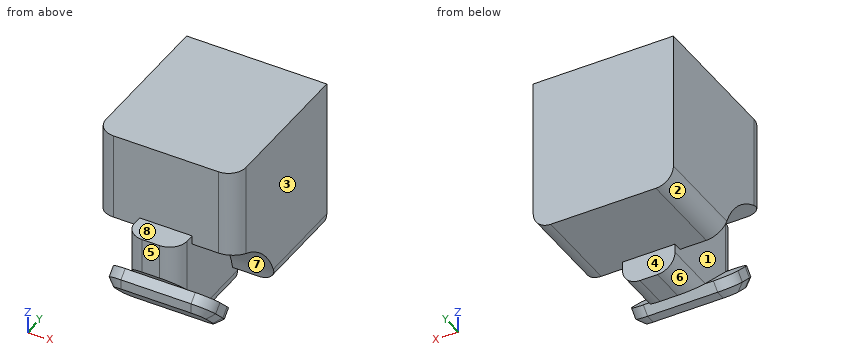
```python
from build123d import *

# Parameters (mm, degrees)
F0_W     = 40
F0_H     = 45
F1_DEPTH = 22.5
F3_DEPTH = 40.001
F5_DEPTH = 7.5
F6_R     = 5
F7_W     = 30
F7_H     = 15
F8_DEPTH = 5
F9_R     = 5
F10_SIZE = 2


with BuildPart() as f1:
    # F0 (on Top) → F1 (new body, symmetric)
    with BuildSketch(Plane.XY):
        Rectangle(F0_W, F0_H)
    extrude(amount=F1_DEPTH, both=True)

    # F2 (on face) → F3 (cut, through all)
    with BuildSketch(Plane(origin=(-20, 0, 0), x_dir=(0, -1, 0), z_dir=(-1, 0, 0))):
        with BuildLine():
            Line((2.5, -22.5), (22.5, -22.5))
            Line((22.5, -22.5), (22.5, -2.5))
            ThreePointArc((22.5, -2.5), (9.39971, -9.39971), (2.5, -22.5))
        make_face()
    extrude(amount=-F3_DEPTH, mode=Mode.SUBTRACT)

    # F4 (on Right) → F5 (join, symmetric)
    with BuildSketch(Plane.YZ):
        Polygon((0, -30), (0, 0), (-30, 0), (-30, -10), (-10, -30), align=None)
    extrude(amount=F5_DEPTH, both=True)

    # F6
    f6_edges = [f1.edges().sort_by_distance(p)[0] for p in [
        (-20, -22.5, 10),
        (20, -22.5, 10),
        (-20, 10, -22.5),
        (20, 10, -22.5),
        (7.5, -30, -5),
        (-7.5, -30, -5),
        (7.5, -5, -30),
        (-7.5, -5, -30),
    ]]
    fillet(f6_edges, radius=F6_R)

    # F7 (on face) → F8 (join)
    with BuildSketch(Plane(origin=(0, -20, -20), x_dir=(1, 0, 0), z_dir=(0, -0.707107, -0.707107))):
        Rectangle(F7_W, F7_H)
    extrude(amount=F8_DEPTH)

    # F9
    f9_edges = [f1.edges().sort_by_distance(p)[0] for p in [
        (-15, -27.071068, -16.464466),
        (-15, -16.464466, -27.071068),
        (15, -16.464466, -27.071068),
        (15, -27.071068, -16.464466),
    ]]
    fillet(f9_edges, radius=F9_R)

    # F10
    f10_edges = [f1.edges().sort_by_distance(p)[0] for p in [
        (0, -18.232233, -28.838835),
    ]]
    chamfer(f10_edges, length=F10_SIZE)


solid = f1.part
```
Build history of the part. All positions in model axes, mm. Face numbers are marked on the shaded views. A direction names the side the tool comes from. Give positions to 0.01 mm unless a question says otherwise; leave off trailing zeros. Order: outer loops, then holes, each group sorted by start corner. A loop starts at its lowest first (then second) coordinate and runs counter-clockwise, first axis right, second up. Notation, with made-up numbers: M -21,88.5 L -1,88.5 A26 cw -1,125.5 Z; hole C -2.5,18.25 d8. An arc over 180 degrees is marked long. Write item = value, one per line. Start each with the question number.
(1) Slice it at D-D on z = 15.5. Write the cut outline in (x, y).
(2) Two-plate mould, pull along Z, no slides. Class the marked faces 1, 2 and 3: released by +Z, released by -Z, zero draft, split by the parting line, or undercut.
(3) Probe L1, parallel to Y at x = 0, z = 0.5; L2, parallel to Z at x = -5, y = -27; L3, parallel to Z at x = 0, y = -25.5. List the from-to ranges inside material, lowest first. Write a range as [from, to].
(4) Which spindle directions (+Z, -Z, +X, -X, +Y, -Y) get a long thin tool onto all of the face, cutting with end or side? Do the marked faces 4, 5, 6, 7 and 8. Say none if no direction does.
(5) Slice it at B-B on y = -12. Write the cut outline in (x, z), plus the area to 3 significant figures.
(6) Slice it at C-C on x = -6. Write the cut outline in (y, z).
(7) Slice it at A-A on z = -13. Write the cut outline in (x, y).
(8) Pin check, flat tips, straight feed: pin 1 Ø20 at (y, z) = (-11, -9.5) entering from +X; pin 2 Ø6 at (x, z) = (0.5, -26) entering from +Y; pin 3 Ø7.5 at (x, z) = (-1.5, 8) entering from -Y; pin 4 Ø10 at (x, y) = (15.5, -16) entering from -Z. Stop position of each tip, or through.
Responses:
q1.outline = M -20,-17.5 A5 ccw -15,-22.5 L 15,-22.5 A5 ccw 20,-17.5 L 20,22.5 L -20,22.5 Z
q2.face_1 = undercut
q2.face_2 = released by -Z
q2.face_3 = zero draft
q3.L1 = [-22.5, 22.5]
q3.L2 = [-20.07, -16.39], [-13, 0]
q3.L3 = [-21.57, -14.89], [-14.5, 0]
q4.face_4 = -Z, +X, -X, +Y
q4.face_5 = +Z, -Z, +X, -X, -Y
q4.face_6 = -Z, -X, +Y
q4.face_7 = +X
q4.face_8 = +Z, +X, -X, -Y
q5.outline = M -20,-7.14 L -7.5,-7.14 L -7.5,-25 A5 ccw -6.5,-28 L 6.5,-28 A5 ccw 7.5,-25 L 7.5,-7.14 L 20,-7.14 L 20,22.5 L -20,22.5 Z
q5.area = 1,500 mm2
q6.outline = M -28.57,-11.43 L -25.3,-14.7 L -27.42,-16.82 L -27.42,-19.65 L -19.65,-27.42 L -16.82,-27.42 L -14.7,-25.3 L -11.43,-28.57 L 0,-28.57 L 0,-22.5 L 22.5,-22.5 L 22.5,22.5 L -22.5,22.5 L -22.5,0 L -28.57,0 Z
q7.outline = M -20,-6.42 L -7.5,-6.42 L -7.5,-25 A5 ccw -7.08,-27 L 7.08,-27 A5 ccw 7.5,-25 L 7.5,-6.42 L 20,-6.42 L 20,22.5 L -20,22.5 Z
q8.pin_1 = 20
q8.pin_2 = 0
q8.pin_3 = -22.5
q8.pin_4 = -27.4
